Can you work these out from the drawing? Everything is in mm from the part's minimum corner. Round coordinates to 2 decimals unless told otherwise and drop trailing zeros. Write each loop counter-clockwise with the first axis right and the second up, starting at its lowest first coordinate (ties: lowest second). Pieces come first, ordered by that corner, then holes. Notation, with made-up numbers: M -2,87.5 L 9,87.5 A17 ccw 9,100.5 Z; hole C 69.5,89 d1. An arc over 180 degrees is marked long. Answer in a Markdown table with one row per item. Add a question column.
(1) Suppose I cut it at C-C, the plane x = 4.5. Write out the boundary of the cut face in (y, z), then the cut area to 3 significant figures.
(2) Suppose I cut it at A-A, the plane z = 9. Write out the boundary of the cut face in (x, y), then the cut area to 3 significant figures.
(3) Suppose I cut it at B-B, the plane y = 9. Write out the boundary of the cut face in (x, z), then the cut area to 3 significant figures.
(4) Suppose I cut it at D-D, the plane x = 37. Write out the boundary of the cut face in (y, z), then the cut area to 3 significant figures.
(5) I'm going to push flat-ended pins straight in: pin 1 (4 mm diameter, centred on x = 12.5, y = 5.5, fed in from -Z); pin 2 (2 mm diameter, centred on x = 32.5, z = 2, fed in from +Y); pin 3 (3 mm diameter, centred on x = 35, y = 14, fed in from -Z); pin 4 (2 mm diameter, centred on x = 65.5, y = 9, fed in from +Z). Where does each tip first touch, or does it pass through?
(6) If I drill on probe 1 along Z at (x, y) = (30, 8.5); probe 2 along Y at (x, z) = (22, 2.5); probe 3 along Z at (x, y) = (29.5, 3.75), over which ranges is the centre line in solid material (lowest first)?
(7) If we mould it in two halves opening along Y, with no side actions, what happens to the marked faces 1 and 2? For each: released by +Y, released by -Y, zero draft, split by the parting line, or undercut.
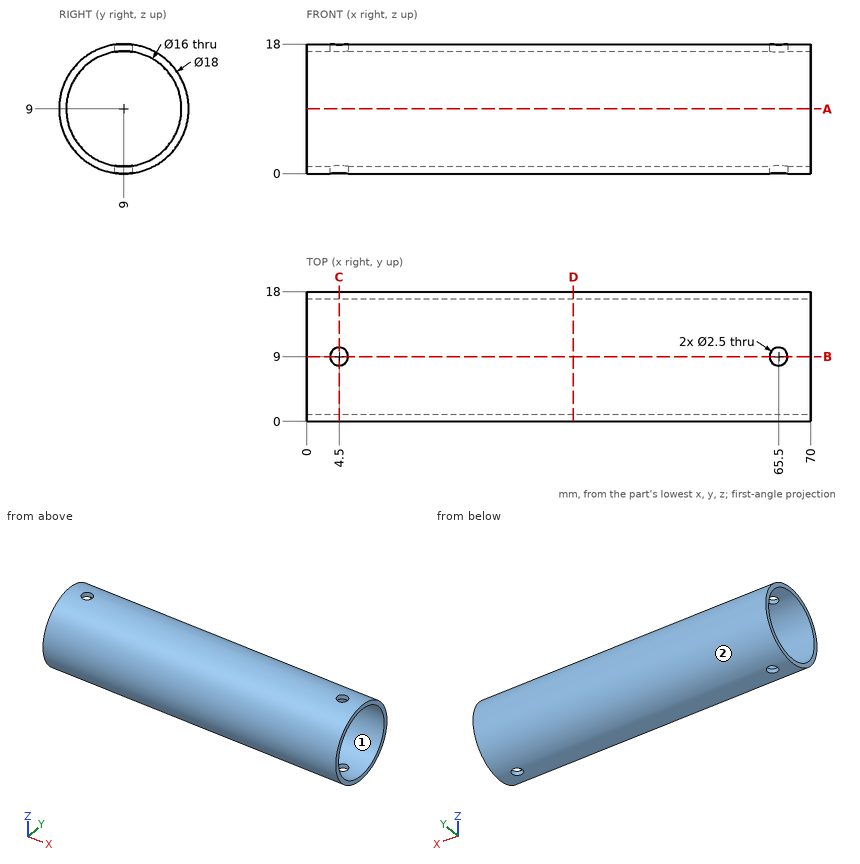
Calculated:
| question | item | result |
|---|---|---|
| 1 | outline | M 7.75,0.09 L 7.75,1.1 A8 cw 7.75,16.9 L 7.75,17.91 A9 ccw Z; M 10.25,0.09 A9 ccw 10.25,17.91 L 10.25,16.9 A8 cw 10.25,1.1 Z |
| 1 | area | 48.4 mm² |
| 2 | outline | M 0,0 L 70,0 L 70,1 L 0,1 Z; M 0,17 L 70,17 L 70,18 L 0,18 Z |
| 2 | area | 140 mm² |
| 3 | outline | M 0,0 L 3.25,0 L 3.25,1 L 0,1 Z; M 0,17 L 3.25,17 L 3.25,18 L 0,18 Z; M 5.75,0 L 64.25,0 L 64.25,1 L 5.75,1 Z; M 5.75,17 L 64.25,17 L 64.25,18 L 5.75,18 Z; M 66.75,0 L 70,0 L 70,1 L 66.75,1 Z; M 66.75,17 L 70,17 L 70,18 L 66.75,18 Z |
| 3 | area | 130 mm² |
| 4 | outline | C 9,9 d18; hole C 9,9 d16 |
| 4 | area | 53.4 mm² |
| 5 | pin 1 | z = 0.13 |
| 5 | pin 2 | y = 15.71 |
| 5 | pin 3 | z = 0.71 |
| 5 | pin 4 | through |
| 6 | probe 1 | 0.01 to 1.02, 16.98 to 17.99 |
| 6 | probe 2 | 2.78 to 4.34, 13.66 to 15.22 |
| 6 | probe 3 | 1.69 to 2.96, 15.04 to 16.31 |
| 7 | face 1 | undercut |
| 7 | face 2 | split by the parting line |
